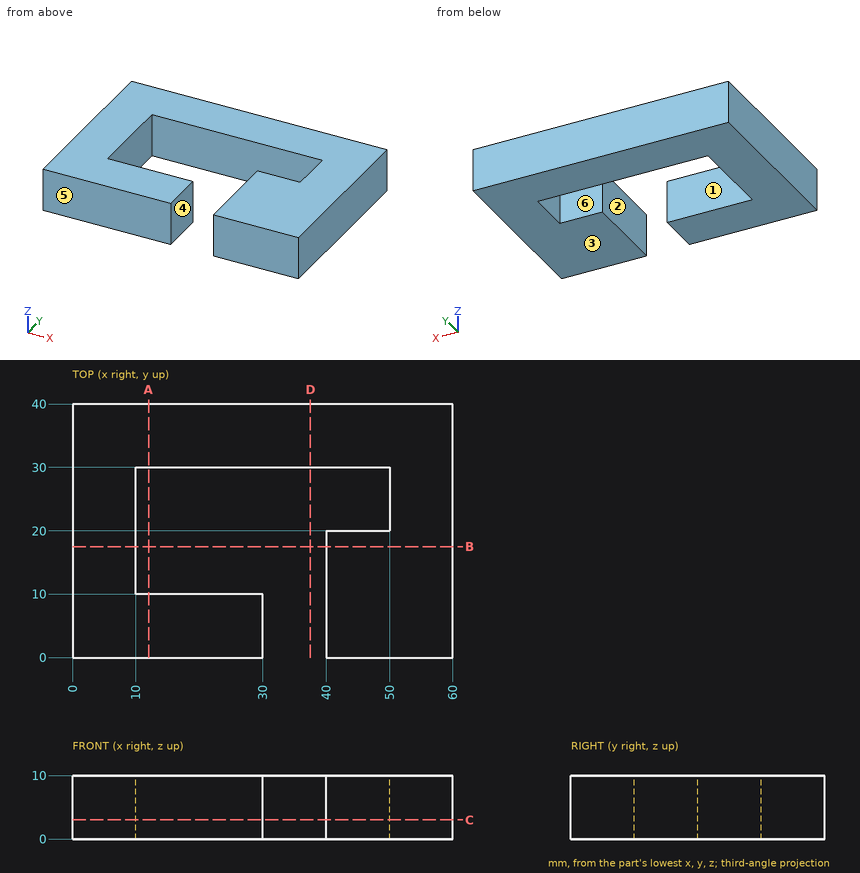
Geometry: see drawing. Coordinates: mm, zero at the bounding-box minimum. A direction names the side the tool comes from. Give positions to 0.01 mm unless a question says otherwise; leave off trailing zeros. Loops run counter-clockwise (first coordinate to the right, second up) from the corner with the lowest first, then second, coordinate; pieces in that order, holes last. Notation, with made-up numbers: (-27.75, 32.5) - (17.25, 32.5) arc R26 cw to (17.25, 55.5) - close; hole circle Ø1 at (-2, -21.75). An arc over 180 degrees is marked (long way). Use CSV: the item, a comma, the result in double quotes. Start each with the question number.
Item 1: Reachability of the marked faces 1, 2 and 3 from +Z, -Z, +X, -X, +Y, -Y: full face, straight path, thin tool, end or side. Return the list, or none.
Item 2: Section C-C on z = 3. Return loops of the section in (x, y).
Item 3: Section B-B on y = 17.5. Return loops of the section in (x, z).
Item 4: Line query: line 1 (X direction, y = 29.5, z = 9); line 2 (X direction, y = 15, z = 8.25); line 3 (Y direction, x = 43.5, z = 4). Output: solid intervals per line, ascending.
Item 5: Mould query, pull axis Y, two halves, no side actions, for the marked faces 4, 5 and 6. Classes: pulls with the +Y half, pulls with the -Y half, needs draft (parallel to the pull), parting line crosses it, or undercut.
Item 6: Contact query for a flat-ended pin moving along its axis: P1, Ø3, axis at x = 34.5, z = 7.5, coming from the -Y side. Output: stop coordinate, or through.
Item 7: Section D-D on x = 37.5. Return loops of the section in (y, z), then the cut area to 3 significant figures.
Item 8: Section A-A on x = 12. Return loops of the section in (y, z), then the cut area to 3 significant figures.
Ans:
1,face 1,"+Z, -Z"
1,face 2,"+Z, -Z, -Y"
1,face 3,"-Z, +X, -X, +Y, -Y"
2,outline,"(0, 0) - (30, 0) - (30, 10) - (10, 10) - (10, 30) - (50, 30) - (50, 20) - (40, 20) - (40, 0) - (60, 0) - (60, 40) - (0, 40) - close"
3,outline,"(0, 0) - (10, 0) - (10, 10) - (0, 10) - close; (40, 0) - (60, 0) - (60, 10) - (40, 10) - close"
4,line 1,"x = 0 to 10, 50 to 60"
4,line 2,"x = 0 to 10, 40 to 60"
4,line 3,"y = 0 to 20, 30 to 40"
5,face 4,"needs draft"
5,face 5,"pulls with the -Y half"
5,face 6,"undercut"
6,P1,"stops at y = 30"
7,outline,"(30, 0) - (40, 0) - (40, 10) - (30, 10) - close"
7,area,"100 mm2"
8,outline,"(0, 0) - (10, 0) - (10, 10) - (0, 10) - close; (30, 0) - (40, 0) - (40, 10) - (30, 10) - close"
8,area,"200 mm2"
